```python
from build123d import *

# Parameters (mm, degrees)
SKETCH1_W                = 102
SKETCH1_H                = 105
BOSS_EXTRUDE1_DEPTH      = 1.5
SKETCH2_W                = 3
SKETCH2_H                = 10
BOSS_EXTRUDE2_DEPTH      = 23
FILLET1_R                = 2
M3_CLEARANCE_HOLE1_D     = 3.4
SKETCH6_W                = 3
SKETCH6_H                = 10
BOSS_EXTRUDE3_DEPTH      = 17
M3_CLEARANCE_HOLE2_D     = 3.4
M3_CLEARANCE_HOLE2_DEPTH = 3
CUT_EXTRUDE1_DEPTH       = 10
SKETCH10_R               = 6
CUT_EXTRUDE2_DEPTH       = 10
FILLET2_R                = 3
FILLET3_R                = 0.5


with BuildPart() as part:
    # Sketch1 → Boss-Extrude1 (new, symmetric)
    with BuildSketch(Plane.XY):
        Rectangle(SKETCH1_W, SKETCH1_H)
    extrude(amount=BOSS_EXTRUDE1_DEPTH, both=True)

    # Sketch2 → Boss-Extrude2 (add)
    with BuildSketch(Plane(origin=(0, 0, -1.5), x_dir=(-1, 0, 0), z_dir=(0, 0, -1))):
        with Locations((42.57, -34.23)):
            Rectangle(SKETCH2_W, SKETCH2_H)
    extrude(amount=BOSS_EXTRUDE2_DEPTH)

    # Fillet1
    fillet1_edges = [part.edges().sort_by_distance(p)[0] for p in [
        (-44.07, -34.23, -1.5),
        (-41.07, -34.23, -1.5),
    ]]
    fillet(fillet1_edges, radius=FILLET1_R)

    # M3 Clearance Hole1 (through all)
    with Locations(Plane.ZY.offset(44.07)):
        with Locations((-20.5, -34.23)):
            Hole(M3_CLEARANCE_HOLE1_D / 2)

    # Sketch6 → Boss-Extrude3 (add)
    with BuildSketch(Plane(origin=(0, 0, -1.5), x_dir=(-1, 0, 0), z_dir=(0, 0, -1))):
        with Locations((-49.5, -37.5)):
            Rectangle(SKETCH6_W, SKETCH6_H)
    boss_extrude3 = extrude(amount=BOSS_EXTRUDE3_DEPTH)

    # M3 Clearance Hole2
    with Locations(Plane(origin=(51, 0, 0), x_dir=(0, 0, -1), z_dir=(1, 0, 0))):
        with Locations((13.5, -37.5)):
            m3_clearance_hole2 = Hole(M3_CLEARANCE_HOLE2_D / 2, depth=M3_CLEARANCE_HOLE2_DEPTH)

    # Sketch9 → Cut-Extrude1 (cut)
    with BuildSketch(Plane.XY.offset(1.5)):
        with BuildLine():
            Line((-20, 6), (20, 6))
            ThreePointArc((20, 6), (21, 5), (20, 4))
            Line((20, 4), (-20, 4))
            ThreePointArc((-20, 4), (-21, 5), (-20, 6))
        make_face()
        with BuildLine():
            Line((-20, 1), (20, 1))
            ThreePointArc((20, 1), (21, 0), (20, -1))
            Line((20, -1), (-20, -1))
            ThreePointArc((-20, -1), (-21, 0), (-20, 1))
        make_face()
        with BuildLine():
            Line((-20, -4), (20, -4))
            ThreePointArc((20, -4), (21, -5), (20, -6))
            Line((20, -6), (-20, -6))
            ThreePointArc((-20, -6), (-21, -5), (-20, -4))
        make_face()
        with BuildLine():
            Line((-20, 11), (20, 11))
            ThreePointArc((20, 11), (21, 10), (20, 9))
            Line((20, 9), (-20, 9))
            ThreePointArc((-20, 9), (-21, 10), (-20, 11))
        make_face()
        with BuildLine():
            Line((-20, -9), (20, -9))
            ThreePointArc((20, -9), (21, -10), (20, -11))
            Line((20, -11), (-20, -11))
            ThreePointArc((-20, -11), (-21, -10), (-20, -9))
        make_face()
        with BuildLine():
            Line((-20, 16), (20, 16))
            ThreePointArc((20, 16), (21, 15), (20, 14))
            Line((20, 14), (-20, 14))
            ThreePointArc((-20, 14), (-21, 15), (-20, 16))
        make_face()
        with BuildLine():
            Line((-20, 21), (20, 21))
            ThreePointArc((20, 21), (21, 20), (20, 19))
            Line((20, 19), (-20, 19))
            ThreePointArc((-20, 19), (-21, 20), (-20, 21))
        make_face()
        with BuildLine():
            Line((-20, -14), (20, -14))
            ThreePointArc((20, -14), (21, -15), (20, -16))
            Line((20, -16), (-20, -16))
            ThreePointArc((-20, -16), (-21, -15), (-20, -14))
        make_face()
        with BuildLine():
            Line((-20, -19), (20, -19))
            ThreePointArc((20, -19), (21, -20), (20, -21))
            Line((20, -21), (-20, -21))
            ThreePointArc((-20, -21), (-21, -20), (-20, -19))
        make_face()
    extrude(amount=-CUT_EXTRUDE1_DEPTH, mode=Mode.SUBTRACT)

    # Sketch10 → Cut-Extrude2 (cut)
    with BuildSketch(Plane(origin=(0, 0, -1.5), x_dir=(-1, 0, 0), z_dir=(0, 0, -1))):
        with Locations((0, -37.5)):
            Circle(SKETCH10_R)
    extrude(amount=-CUT_EXTRUDE2_DEPTH, mode=Mode.SUBTRACT)

    # Mirror1: Boss-Extrude3, M3 Clearance Hole2 across plane
    add(boss_extrude3.mirror(Plane.ZX))
    add(m3_clearance_hole2.mirror(Plane.ZX), mode=Mode.SUBTRACT)

    # Fillet2
    fillet2_edges = [part.edges().sort_by_distance(p)[0] for p in [
        (49.5, -32.5, -1.5),
    ]]
    fillet(fillet2_edges, radius=FILLET2_R)
    fillet2_2_edges = [part.edges().sort_by_distance(p)[0] for p in [
        (48, -37.5, -1.5),
    ]]
    fillet(fillet2_2_edges, radius=FILLET2_R)
    fillet2_3_edges = [part.edges().sort_by_distance(p)[0] for p in [
        (49.5, -42.5, -1.5),
    ]]
    fillet(fillet2_3_edges, radius=FILLET2_R)
    fillet2_4_edges = [part.edges().sort_by_distance(p)[0] for p in [
        (49.5, 42.5, -1.5),
    ]]
    fillet(fillet2_4_edges, radius=FILLET2_R)
    fillet2_5_edges = [part.edges().sort_by_distance(p)[0] for p in [
        (48, 37.5, -1.5),
    ]]
    fillet(fillet2_5_edges, radius=FILLET2_R - 0.0001)  # a hair under: the kernel refuses the full size
    fillet2_6_edges = [part.edges().sort_by_distance(p)[0] for p in [
        (49.5, 32.5, -1.5),
    ]]
    fillet(fillet2_6_edges, radius=FILLET2_R - 0.0001)  # a hair under: the kernel refuses the full size
    fillet2_7_edges = [part.edges().sort_by_distance(p)[0] for p in [
        (-42.57, -29.23, -1.5),
    ]]
    fillet(fillet2_7_edges, radius=FILLET2_R)
    fillet2_8_edges = [part.edges().sort_by_distance(p)[0] for p in [
        (-42.57, -39.23, -1.5),
    ]]
    fillet(fillet2_8_edges, radius=FILLET2_R)

    # Fillet3
    fillet3_edges = [part.edges().sort_by_distance(p)[0] for p in [
        (6, -37.5, 1.5),
        (6, -37.5, -1.5),
    ]]
    fillet(fillet3_edges, radius=FILLET3_R)


solid = part.part
```
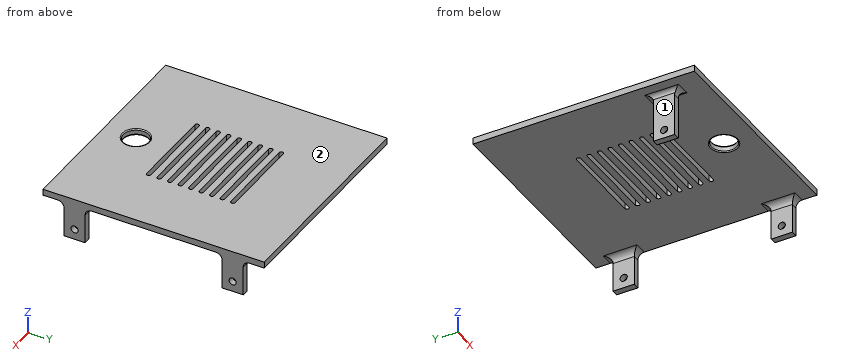
Part model, mm, in its own coordinate system. Face numbers are marked on the shaded views. A direction names the side the tool comes from. Coordinates: 2 decimals unless noted, no trailing zeros. Order: outer loops, then holes, each group sorted by start corner. A loop starts at its lowest first (then second) coordinate and runs counter-clockwise, first axis right, second up. Notation, with made-up numbers: (-19.75, 21) - (32.25, 21) arc R7 ccw to (32.25, 25) - close; hole circle Ø6 at (11.5, 62.25). An arc over 180 degrees is marked (long way). Return JSON: item names as keys, results as strings. Group by question number.
Item 1: Cut at D-D (z = -6.75). List the corners of the cut face in (x, y).
Item 2: Pin check, flat tips, straight feed: pin 1 (2 mm diameter, centred on y = 41.5, z = -16, fed in from -X); pin 2 (5 mm diameter, centred on x = 15, z = -6, fed in from +Y); pin 3 (11.5 mm diameter, centred on y = -33, z = -19, fed in from -X); pin 4 (1.5 mm diameter, centred on x = 49.5, z = -13.5, fed in from -Y). Stop position of each tip, or through.
Item 3: Drill centre lines: probe 1 along Y at (x, z) = (-41.65, -20.5); probe 2 along X at (y, z) = (-38, -8.5); probe 3 along Z at (x, y) = (29, -1.5). Where is each one in solid material? Low to high. Write a range as from..to.
Item 4: Cut at B-B (z = -13.5). List the corners of the cut face in (x, y), plus the area to 3 significant figures.
Item 5: Cut at C-C (y = 37.5). List the corners of the cut face in (x, z), plus the area to 3 significant figures.
Item 6: Cut at A-A (y = -37.5). List the corners of the cut face in (x, z), plus the area to 3 significant figures.
Item 7: Which spindle directions (+Z, -Z, +X, -X, +Y, -Y) get a long thin tool onto all of the face, cutting with end or side? Do the marked faces 1 and 2. Say none if no direction does.
Check values:
{
 "1": {"outline": "(-44.07, -39.23) - (-41.07, -39.23) - (-41.07, -29.23) - (-44.07, -29.23) - close; (48, -42.5) - (51, -42.5) - (51, -32.5) - (48, -32.5) - close; (48, 32.5) - (51, 32.5) - (51, 42.5) - (48, 42.5) - close"},
 "2": {"pin 1": "stops at x = 48", "pin 2": "passes through", "pin 3": "stops at x = -44.07", "pin 4": "stops at y = -42.5"},
 "3": {"probe 1": "y = -39.23..-35.93, -32.53..-29.23", "probe 2": "x = -44.07..-41.07, 48..51", "probe 3": "z = -1.5..1.5"},
 "4": {"outline": "(-44.07, -39.23) - (-41.07, -39.23) - (-41.07, -29.23) - (-44.07, -29.23) - close; (48, -42.5) - (51, -42.5) - (51, -39.2) - (48, -39.2) - close; (48, -35.8) - (51, -35.8) - (51, -32.5) - (48, -32.5) - close; (48, 32.5) - (51, 32.5) - (51, 35.8) - (48, 35.8) - close; (48, 39.2) - (51, 39.2) - (51, 42.5) - (48, 42.5) - close", "area": "69.6 mm2"},
 "5": {"outline": "(-51, -1.5) - (45, -1.5) arc R3 cw to (48, -4.5) - (48, -11.8) - (51, -11.8) - (51, 1.5) - (-51, 1.5) - close; (48, -18.5) - (51, -18.5) - (51, -15.2) - (48, -15.2) - close", "area": "349 mm2"},
 "6": {"outline": "(-51, -1.5) - (-46.07, -1.5) arc R2 cw to (-44.07, -3.5) - (-44.07, -24.5) - (-41.07, -24.5) - (-41.07, -3.5) arc R2 cw to (-39.07, -1.5) - (-6.5, -1.5) arc R0.5 ccw to (-6, -1) - (-6, 1) arc R0.5 ccw to (-6.5, 1.5) - (-51, 1.5) - close; (6, -1) arc R0.5 ccw to (6.5, -1.5) - (45, -1.5) arc R3 cw to (48, -4.5) - (48, -11.8) - (51, -11.8) - (51, 1.5) - (6.5, 1.5) arc R0.5 ccw to (6, 1) - close; (48, -18.5) - (51, -18.5) - (51, -15.2) - (48, -15.2) - close", "area": "383 mm2"},
 "7": {"face 1": "-Z, -X, +Y, -Y", "face 2": "+Z, +X, -X, +Y, -Y"}
}
